```python
from build123d import *

# Parameters (mm, degrees)
F0_W     = 120
F0_H     = 122
F0_H_2   = 76
F1_DEPTH = 10
F3_D     = 4.2
F5_D     = 4.2
F7_D     = 4.2
F7_DEPTH = 12.4
F7_TIP   = 1.2618073


# Not quite as in the source:
# - a feature names something its author has since deleted; it is built from what else it names


with BuildPart() as f1:
    # F0 (on Front) → F1 (new body)
    with BuildSketch(Plane.XZ):
        Rectangle(F0_W, F0_H)
        with Locations((0, 99)):
            Rectangle(F0_W, F0_H_2)
    extrude(amount=F1_DEPTH)

    # F3 (through all)
    with Locations(Plane(origin=(0, 0, 0), x_dir=(-1, 0, 0), z_dir=(0, 1, 0))):
        with Locations((-55, 55.25), (-29, 55.25), (-29, 24.75), (-55, 24.75), (29, 55.25), (55, 55.25), (55, 24.75), (29, 24.75), (-13, -24.75), (13, -24.75), (13, -55.25), (-13, -55.25), (0, 10), (0, -10)):
            Hole(F3_D / 2)

    # F5 (through all)
    with Locations(Plane(origin=(0, 0, 0), x_dir=(-1, 0, 0), z_dir=(0, 1, 0))):
        with Locations((-55.25, 130), (-23.25, 130), (23.25, 130), (55.25, 130), (-55.25, -54), (-23.25, -54), (23.25, -54), (55.25, -54)):
            Hole(F5_D / 2)

    # F7
    with Locations(Plane.XY.offset(137)):
        with Locations((11, -5), (-11, -5)):
            Hole(F7_D / 2, depth=F7_DEPTH)
            with Locations((0, 0, -(F7_DEPTH + F7_TIP / 2))):  # 118° drill point
                Cone(0, F7_D / 2, F7_TIP, mode=Mode.SUBTRACT)


solid = f1.part
```
Geometry: final body of the model. Coordinates: model frame, mm. Give positions to 0.01 mm unless a question says otherwise; leave off trailing zeros. Write each loop counter-clockwise with the first axis right and the second up, starting at its lowest first coordinate (ties: lowest second). Pieces come first, ordered by that corner, then holes.
1. Section query B-B, the plane x = 29. Return loops of the section in (y, z), then the cut area to 3 significant figures.
2. Draft query along Y for faces 1 (the flat face through (-1, -10, 39)), 2 (the flat face through (-60, -5, 39)), 3 (the cylindrical face through (12.666, -6.278, 130.713)). Return one class per face: released by +Y, released by -Y, zero draft, split by the parting line, or undercut.
3. Line query: probe 1 along Z at (x, y) = (-55, -7.25); probe 2 along Z at (x, y) = (-23.25, -7.75); probe 3 along Z at (x, y) = (0, -2.75). Output: solid intervals per line, ascending.
4. Pin query (flat end, axial travel): P1, Ø3.5, axis at x = 11, y = -5, coming from the +Z side. Return the tip coordinate at first contact, or that it passes through.
5. Section query A-A, the plane z = -10. Return loops of the section in (x, y), then the cut area to 3 significant figures.
Computed:
1. outline: (-10, -61) - (0, -61) - (0, 22.65) - (-10, 22.65) - close; (-10, 26.85) - (0, 26.85) - (0, 53.15) - (-10, 53.15) - close; (-10, 57.35) - (0, 57.35) - (0, 137) - (-10, 137) - close
1. area: 1,900 mm2
2. face 1: released by -Y
2. face 2: zero draft
2. face 3: undercut
3. probe 1: z = -61 to -56.09, -51.91 to 22.65, 26.85 to 53.15, 57.35 to 127.91, 132.09 to 137
3. probe 2: z = -61 to -56.1, -51.9 to 127.9, 132.1 to 137
3. probe 3: z = -61 to -12.1, -7.9 to 7.9, 12.1 to 137
4. P1: stops at z = 124.39
5. outline: (-60, -10) - (-2.1, -10) - (-2.1, 0) - (-60, 0) - close; (2.1, -10) - (60, -10) - (60, 0) - (2.1, 0) - close
5. area: 1,160 mm2
